Here's how the part is built. I have some questions about the finished solid (model axes, mm). Face numbers are marked on the shaded views. Round coordinates to 2 decimals unless told otherwise and drop trailing zeros. Loops run counter-clockwise (first coordinate to the right, second up) from the corner with the lowest first, then second, coordinate; pieces in that order, holes last. Notation, with made-up numbers: M 63.5,88.5 L 81.5,88.5 A27 ccw 81.5,122.5 Z; hole C 41,70.5 d1. An arc over 180 degrees is marked long. Use a Markdown table: item, result.
from build123d import *

# Parameters (mm, degrees)
SKETCH1_R               = 19.5
SKETCH1_R_2             = 6
SKETCH1_R_3             = 2.5
SKETCH1_R_4             = 2
BOSS_EXTRUDE1_DEPTH     = 6
SKETCH5_R               = 2
BOSS_EXTRUDE2_DEPTH     = 5.5
CUT_EXTRUDE2_DEPTH      = 4
CHAMFER1_SIZE           = 1
CHAMFER2_SIZE           = 0.5
CUT_EXTRUDE3_DEPTH      = 113.093142074
CUT_EXTRUDE3_DEPTH_BACK = 113.093142074
SKETCH8_R               = 0.875
CUT_EXTRUDE4_DEPTH      = 4


with BuildPart() as part:
    # Sketch1 → Boss-Extrude1 (new body)
    with BuildSketch(Plane(origin=(0, 0, 0), x_dir=(1, 0, 0), z_dir=(0, 1, 0))):
        with BuildLine():
            Line((0, 36.25), (67.5, 36.25))
            ThreePointArc((67.5, 36.25), (82.21405629, 33.129428723), (94.394801605, 24.30498193))
            ThreePointArc((94.394801605, 24.30498193), (104.860213633, 20.548117498), (102.428678881, 9.697932337))
            ThreePointArc((102.428678881, 9.697932337), (103.75, 0), (102.428678881, -9.697932337))
            ThreePointArc((102.428678881, -9.697932337), (104.860213633, -20.548117498), (94.394801605, -24.30498193))
            ThreePointArc((94.394801605, -24.30498193), (82.21405629, -33.129428723), (67.5, -36.25))
            Line((67.5, -36.25), (0, -36.25))
            ThreePointArc((0, -36.25), (-14.71405629, -33.129428723), (-26.894801605, -24.30498193))
            ThreePointArc((-26.894801605, -24.30498193), (-37.360213633, -20.548117498), (-34.928678881, -9.697932337))
            ThreePointArc((-34.928678881, -9.697932337), (-36.25, 0), (-34.928678881, 9.697932337))
            ThreePointArc((-34.928678881, 9.697932337), (-37.360213633, 20.548117498), (-26.894801605, 24.30498193))
            ThreePointArc((-26.894801605, 24.30498193), (-14.71405629, 33.129428723), (0, 36.25))
        make_face()
        with Locations(Location((0, 0, 0), (0, 0, 270))):
            Circle(SKETCH1_R, mode=Mode.SUBTRACT)
        with Locations(Location((67.5, 0, 0), (0, 0, 270))):
            Circle(SKETCH1_R_2, mode=Mode.SUBTRACT)
        with Locations(Location((67.5, 18.5, 0), (0, 0, 270))):
            Circle(SKETCH1_R_3, mode=Mode.SUBTRACT)
        with Locations(Location((67.5, -18.5, 0), (0, 0, 270))):
            Circle(SKETCH1_R_3, mode=Mode.SUBTRACT)
        with Locations(Location((-30, 16.5, 0), (0, 0, 270))):
            Circle(SKETCH1_R_4, mode=Mode.SUBTRACT)
        with Locations(Location((-30, -16.5, 0), (0, 0, 270))):
            Circle(SKETCH1_R_4, mode=Mode.SUBTRACT)
        with Locations(Location((97.5, -16.5, 0), (0, 0, 270))):
            Circle(SKETCH1_R_4, mode=Mode.SUBTRACT)
        with Locations(Location((97.5, 16.5, 0), (0, 0, 270))):
            Circle(SKETCH1_R_4, mode=Mode.SUBTRACT)
    extrude(amount=BOSS_EXTRUDE1_DEPTH)

    # Sketch5 → Boss-Extrude2 (add)
    with BuildSketch(Plane(origin=(0, 6, 0), x_dir=(1, 0, 0), z_dir=(0, 1, 0))):
        with BuildLine():
            Line((0, 36.25), (67.5, 36.25))
            ThreePointArc((67.5, 36.25), (82.21405629, 33.129428723), (94.394801605, 24.30498193))
            ThreePointArc((94.394801605, 24.30498193), (104.860213633, 20.548117498), (102.428678881, 9.697932337))
            ThreePointArc((102.428678881, 9.697932337), (103.75, 0), (102.428678881, -9.697932337))
            ThreePointArc((102.428678881, -9.697932337), (104.860213633, -20.548117498), (94.394801605, -24.30498193))
            ThreePointArc((94.394801605, -24.30498193), (82.21405629, -33.129428723), (67.5, -36.25))
            Line((67.5, -36.25), (0, -36.25))
            ThreePointArc((0, -36.25), (-14.71405629, -33.129428723), (-26.894801605, -24.30498193))
            ThreePointArc((-26.894801605, -24.30498193), (-37.360213633, -20.548117498), (-34.928678881, -9.697932337))
            ThreePointArc((-34.928678881, -9.697932337), (-36.25, 0), (-34.928678881, 9.697932337))
            ThreePointArc((-34.928678881, 9.697932337), (-37.360213633, 20.548117498), (-26.894801605, 24.30498193))
            ThreePointArc((-26.894801605, 24.30498193), (-14.71405629, 33.129428723), (0, 36.25))
        make_face()
        with Locations(Location((-30, 16.5, 0), (0, 0, 270))):
            Circle(SKETCH5_R, mode=Mode.SUBTRACT)
        with Locations(Location((97.5, 16.5, 0), (0, 0, 270))):
            Circle(SKETCH5_R, mode=Mode.SUBTRACT)
        with Locations(Location((97.5, -16.5, 0), (0, 0, 270))):
            Circle(SKETCH5_R, mode=Mode.SUBTRACT)
        with Locations(Location((-30, -16.5, 0), (0, 0, 270))):
            Circle(SKETCH5_R, mode=Mode.SUBTRACT)
        with BuildLine():
            Line((0, 33.25), (67.5, 33.25))
            ThreePointArc((67.5, 33.25), (82.073642664, 29.885973959), (93.698346174, 20.474597865))
            ThreePointArc((93.698346174, 20.474597865), (92.680812502, 13.849446876), (98.820847684, 11.160958757))
            ThreePointArc((98.820847684, 11.160958757), (100.75, 0), (98.820847684, -11.160958757))
            ThreePointArc((98.820847684, -11.160958757), (92.680812502, -13.849446876), (93.698346174, -20.474597865))
            ThreePointArc((93.698346174, -20.474597865), (82.073642664, -29.885973959), (67.5, -33.25))
            Line((67.5, -33.25), (0, -33.25))
            ThreePointArc((0, -33.25), (-14.573642664, -29.885973959), (-26.198346174, -20.474597865))
            ThreePointArc((-26.198346174, -20.474597865), (-25.180812502, -13.849446876), (-31.320847684, -11.160958757))
            ThreePointArc((-31.320847684, -11.160958757), (-33.25, 0), (-31.320847684, 11.160958757))
            ThreePointArc((-31.320847684, 11.160958757), (-25.180812502, 13.849446876), (-26.198346174, 20.474597865))
            ThreePointArc((-26.198346174, 20.474597865), (-14.573642664, 29.885973959), (0, 33.25))
        make_face(mode=Mode.SUBTRACT)
    extrude(amount=BOSS_EXTRUDE2_DEPTH)

    # Sketch6 → Cut-Extrude2 (cut)
    with BuildSketch(Plane(origin=(0, 11.5, 0), x_dir=(1, 0, 0), z_dir=(0, 1, 0))):
        Polygon((-25.843078062, 16.5), (-27.921539031, 20.1), (-32.078460969, 20.1), (-34.156921938, 16.5), (-32.078460969, 12.9), (-27.921539031, 12.9), align=None)
        Polygon((-34.156921938, -16.5), (-32.078460969, -20.1), (-27.921539031, -20.1), (-25.843078062, -16.5), (-27.921539031, -12.9), (-32.078460969, -12.9), align=None)
        Polygon((101.656921938, 16.5), (99.578460969, 20.1), (95.421539031, 20.1), (93.343078062, 16.5), (95.421539031, 12.9), (99.578460969, 12.9), align=None)
        Polygon((99.578460969, -20.1), (101.656921938, -16.5), (99.578460969, -12.9), (95.421539031, -12.9), (93.343078062, -16.5), (95.421539031, -20.1), align=None)
    extrude(amount=-CUT_EXTRUDE2_DEPTH, mode=Mode.SUBTRACT)

    # Chamfer1
    chamfer1_edges = [part.edges().sort_by_distance(p)[0] for p in [
        (-14.71405629, 0, -33.129428723),
        (33.75, 0, -36.25),
        (82.21405629, 0, -33.129428723),
        (104.860213633, 0, -20.548117498),
        (103.75, 0, 0),
        (104.860213633, 0, 20.548117498),
        (82.21405629, 0, 33.129428723),
        (33.75, 0, 36.25),
        (-14.71405629, 0, 33.129428723),
        (-37.360213633, 0, 20.548117498),
        (-36.25, 0, 0),
        (-37.360213633, 0, -20.548117498),
        (-14.71405629, 11.5, 33.129428723),
        (33.75, 11.5, 36.25),
        (82.21405629, 11.5, 33.129428723),
        (104.860213633, 11.5, 20.548117498),
        (103.75, 11.5, 0),
        (104.860213633, 11.5, -20.548117498),
        (82.21405629, 11.5, -33.129428723),
        (33.75, 11.5, -36.25),
        (-14.71405629, 11.5, -33.129428723),
        (-37.360213633, 11.5, -20.548117498),
        (-36.25, 11.5, 0),
        (-37.360213633, 11.5, 20.548117498),
        (100.75, 11.5, 0),
        (82.073642664, 11.5, -29.885973959),
        (33.75, 11.5, -33.25),
        (-14.573642664, 11.5, -29.885973959),
        (-33.25, 11.5, 0),
        (-14.573642664, 11.5, 29.885973959),
        (33.75, 11.5, 33.25),
        (82.073642664, 11.5, 29.885973959),
    ]]
    chamfer(chamfer1_edges, length=CHAMFER1_SIZE)

    # Chamfer2
    chamfer2_edges = [part.edges().sort_by_distance(p)[0] for p in [
        (-30, 11.5, -12.9),
        (-33.117691454, 11.5, -14.7),
        (-33.117691454, 11.5, -18.3),
        (-30, 11.5, -20.1),
        (-26.882308546, 11.5, -14.7),
        (-26.882308546, 11.5, -18.3),
        (-25.180812502, 11.5, -13.849446876),
        (-30, 11.5, 20.1),
        (-33.117691454, 11.5, 18.3),
        (-33.117691454, 11.5, 14.7),
        (-30, 11.5, 12.9),
        (-26.882308546, 11.5, 18.3),
        (-26.882308546, 11.5, 14.7),
        (-25.180812502, 11.5, 13.849446876),
        (100.617691454, 11.5, 18.3),
        (97.5, 11.5, 20.1),
        (94.382308546, 11.5, 18.3),
        (94.382308546, 11.5, 14.7),
        (97.5, 11.5, 12.9),
        (100.617691454, 11.5, 14.7),
        (92.680812502, 11.5, 13.849446876),
        (92.680812502, 11.5, -13.849446876),
        (97.5, 11.5, -12.9),
        (94.382308546, 11.5, -14.7),
        (94.382308546, 11.5, -18.3),
        (97.5, 11.5, -20.1),
        (100.617691454, 11.5, -14.7),
        (100.617691454, 11.5, -18.3),
    ]]
    chamfer(chamfer2_edges, length=CHAMFER2_SIZE)

    # Sketch8 → Cut-Extrude3 (cut, two sides: drawn at the far end of the back side and taken through both)
    with BuildSketch(Plane(origin=(0, 6, 0), x_dir=(1, 0, 0), z_dir=(0, 1, 0)).offset(-CUT_EXTRUDE3_DEPTH_BACK)):
        with Locations(Location((67.5, 9.525, 0), (0, 0, 270))):
            Circle(SKETCH8_R)
        with Locations(Location((67.5, -9.525, 0), (0, 0, 270))):
            Circle(SKETCH8_R)
    extrude(amount=CUT_EXTRUDE3_DEPTH + CUT_EXTRUDE3_DEPTH_BACK, mode=Mode.SUBTRACT)

    # Sketch9 → Cut-Extrude4 (cut)
    with BuildSketch(Plane(origin=(0, 6, 0), x_dir=(1, 0, 0), z_dir=(0, 1, 0))):
        Polygon((72.292007234, 18.5), (69.896003617, 22.65), (65.103996383, 22.65), (62.707992766, 18.5), (65.103996383, 14.35), (69.896003617, 14.35), align=None)
        Polygon((72.292007234, -18.5), (69.896003617, -14.35), (65.103996383, -14.35), (62.707992766, -18.5), (65.103996383, -22.65), (69.896003617, -22.65), align=None)
    extrude(amount=-CUT_EXTRUDE4_DEPTH, mode=Mode.SUBTRACT)


solid = part.part
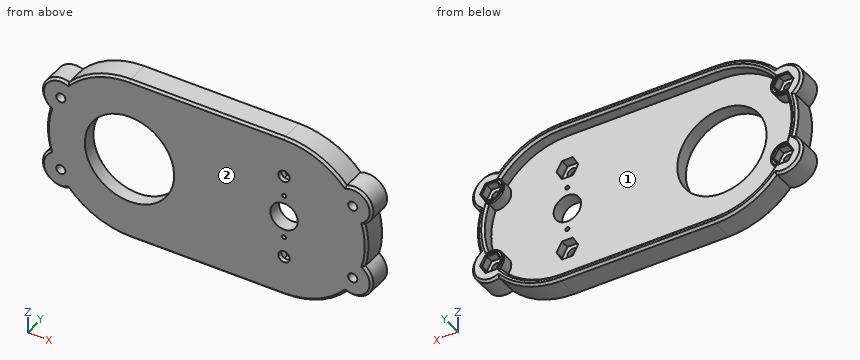
1. Imagine slicing it at B-B, the plane x = 97.5. State how many separate pieces and enclosed holes the cut face has, then the cut area to 3 significant figures.
Answer sheet:
| item | result |
|---|---|
| separate pieces | 3 |
| enclosed holes | 0 |
| area | 331 mm2 |
2. I need wall thicknesses on probe 1 along Z at (x, y) = (97.5, 4); probe 2 along X at (y, z) = (2.75, 0); probe 3 along Z at (x, y) = (47, 7.75). Which ranges of each line are inside material? Lowest first, please. Write a range as from..to.
Answer sheet:
| item | result |
|---|---|
| probe 1 | -24.9..-18.5, -14.5..14.5, 18.5..24.9 |
| probe 2 | -36.25..-19.5, 19.5..61.5, 73.5..103.75 |
| probe 3 | -36.25..-33.25, 33.25..36.25 |
3. Imagine slicing it at C-C, the plane x = 46.5. Write out the boundary of the cut face in (y, z).
Answer sheet:
| item | result |
|---|---|
| outline | M 0,-35.25 L 1,-36.25 L 10.5,-36.25 L 11.5,-35.25 L 11.5,-34.25 L 10.5,-33.25 L 6,-33.25 L 6,33.25 L 10.5,33.25 L 11.5,34.25 L 11.5,35.25 L 10.5,36.25 L 1,36.25 L 0,35.25 Z |
4. Imagine slicing it at A-A, the plane z = 0. Write out the boundary of the cut face in (x, y), then the cut area to 3 significant figures.
Answer sheet:
| item | result |
|---|---|
| outline | M -36.25,1 L -35.25,0 L -19.5,0 L -19.5,6 L -33.25,6 L -33.25,10.5 L -34.25,11.5 L -35.25,11.5 L -36.25,10.5 Z; M 19.5,0 L 61.5,0 L 61.5,6 L 19.5,6 Z; M 73.5,0 L 102.75,0 L 103.75,1 L 103.75,10.5 L 102.75,11.5 L 101.75,11.5 L 100.75,10.5 L 100.75,6 L 73.5,6 Z |
| area | 564 mm2 |
5. Imagine slicing it at D-D, the plane x = 3. Write out the boundary of the cut face in (y, z), then the cut area to 3 significant figures.
Answer sheet:
| item | result |
|---|---|
| outline | M 0,-35.25 L 1,-36.25 L 10.5,-36.25 L 11.5,-35.25 L 11.5,-34.25 L 10.5,-33.25 L 6,-33.25 L 6,-19.27 L 0,-19.27 Z; M 0,19.27 L 6,19.27 L 6,33.25 L 10.5,33.25 L 11.5,34.25 L 11.5,35.25 L 10.5,36.25 L 1,36.25 L 0,35.25 Z |
| area | 234 mm2 |
6. For pin 1 Ø4 at (x, z) = (16, -13.5) entering from +Y; pin 2 Ø2.5 at (x, z) = (-30, 16.5) entering from +Y; pin 3 Ø1 at (x, y) = (76, 7.5) entering from +Z; pin 4 Ø4 at (x, y) = (-29.5, 9.5) entering from -Z, each with a flat end and sliding along its axis, tell me the tip position at first contact or that it passes through.
Answer sheet:
| item | result |
|---|---|
| pin 1 | y = 6 |
| pin 2 | through |
| pin 3 | z = 35.36 |
| pin 4 | z = -24.9 |
7. We'd pull the mould along X, two halves only. Please class the marked faces 1 and 2: +X half, -X half, draft (parallel to the pull), parting line (faces both ways), or undercut.
Answer sheet:
| item | result |
|---|---|
| face 1 | undercut |
| face 2 | draft |
